```python
from build123d import *

# Parameters (mm, degrees)
SKETCH1_R           = 9.5
SKETCH1_R_2         = 1.6
SKETCH1_R_3         = 0.95
BOSS_EXTRUDE1_DEPTH = 10
SKETCH2_R           = 10
BOSS_EXTRUDE2_DEPTH = 10
SKETCH5_R           = 5.5
CUT_EXTRUDE1_DEPTH  = 1.2


with BuildPart() as part:
    # Sketch1 → Boss-Extrude1 (new body)
    with BuildSketch(Plane.XY):
        Circle(SKETCH1_R)
        Circle(SKETCH1_R_2, mode=Mode.SUBTRACT)
        with Locations((-7.5, 0)):
            Circle(SKETCH1_R_3, mode=Mode.SUBTRACT)
        with Locations((-5.303300859, 5.303300859)):
            Circle(SKETCH1_R_3, mode=Mode.SUBTRACT)
        with Locations((0, 7.5)):
            Circle(SKETCH1_R_3, mode=Mode.SUBTRACT)
        with Locations((5.303300859, 5.303300859)):
            Circle(SKETCH1_R_3, mode=Mode.SUBTRACT)
        with Locations((7.5, 0)):
            Circle(SKETCH1_R_3, mode=Mode.SUBTRACT)
        with Locations((5.303300859, -5.303300859)):
            Circle(SKETCH1_R_3, mode=Mode.SUBTRACT)
        with Locations((0, -7.5)):
            Circle(SKETCH1_R_3, mode=Mode.SUBTRACT)
        with Locations((-5.303300859, -5.303300859)):
            Circle(SKETCH1_R_3, mode=Mode.SUBTRACT)
    extrude(amount=BOSS_EXTRUDE1_DEPTH)

    # Sketch2 → Boss-Extrude2 (add)
    with BuildSketch(Plane.XY.offset(10)):
        with Locations(Location((-2, 0, 0), (0, 0, 69.894490212))):
            Circle(SKETCH2_R)
    extrude(amount=BOSS_EXTRUDE2_DEPTH)

    # Sketch5 → Cut-Extrude1 (cut)
    with BuildSketch(Plane(origin=(0, 0, 0), x_dir=(-1, 0, 0), z_dir=(0, 0, -1))):
        Circle(SKETCH5_R)
    extrude(amount=-CUT_EXTRUDE1_DEPTH, mode=Mode.SUBTRACT)


solid = part.part
```
The listing builds one solid part. Answer for the finished solid, in the listing's coordinates (mm). A direction names the side the tool comes from. Round coordinates to 2 decimals unless told otherwise and drop trailing zeros. Order: outer loops, then holes, each group sorted by start corner. A loop starts at its lowest first (then second) coordinate and runs counter-clockwise, first axis right, second up. Notation, with made-up numbers: (18.5, 15.25) -> (30.5, 15.25) arc R16 ccw to (30.5, 36.25) -> close; hole circle Ø11 at (32.5, 74). An arc over 180 degrees is marked (long way). Answer as CSV lines item,"result".
Q1. Consider line 1 (Y direction, x = 0, z = 6); line 2 (X direction, y = -4.75, z = 4.25); line 3 (X direction, y = -0.75, z = 6.5). Determine where each line is inside the solid, lowest interval first. Write a range as from..to.
Computed values:
line 1,"y = -9.5..-8.45, -6.55..-1.6, 1.6..6.55, 8.45..9.5"
line 2,"x = -8.23..-6.08, -4.53..4.53, 6.08..8.23"
line 3,"x = -9.47..-8.08, -6.92..-1.41, 1.41..6.92, 8.08..9.47"
Q2. Given pin 1 (0.9 mm diameter, centred on x = -7.5, y = 0, fed in from -Z); pin 2 (1 mm diameter, centred on x = -2.5, z = 2.5, fed in from +Y); pin 3 (4 mm diameter, centred on y = -3, z = 10, fed in from -X), each flat-ended and moving along its own axis, determine where each tip first touches the part or whether it passes through.
Computed values:
pin 1,"stops at z = 10"
pin 2,"stops at y = 9.29"
pin 3,"stops at x = -11.95"
Q3. A cutting plane is placed at C-C on x = 2.25. Determine the outline of the cut face in (y, z).
Computed values:
outline,"(-9.23, 0) -> (-5.02, 0) -> (-5.02, 1.2) -> (5.02, 1.2) -> (5.02, 0) -> (9.23, 0) -> (9.23, 10) -> (9.05, 10) -> (9.05, 20) -> (-9.05, 20) -> (-9.05, 10) -> (-9.23, 10) -> close"
Q4. For a pull along Y with two mould halves and no side action, classify faces 1 (the cylindrical face through (-1.27, -0.97, 5.54)), 2 (the flat face through (-10, 0, 10)), 3 (the cylindrical face through (0.986, -9.544, 14.93)) as +Y half, -Y half, draft (parallel to the pull), parting line (faces both ways), or undercut.
Computed values:
face 1,"undercut"
face 2,"draft"
face 3,"parting line"
Q5. A cutting plane is placed at A-A on y = 0. Determine the outline of the cut face in (x, z).
Computed values:
outline,"(-12, 10) -> (-9.5, 10) -> (-9.5, 0) -> (-8.45, 0) -> (-8.45, 10) -> (-6.55, 10) -> (-6.55, 0) -> (-5.5, 0) -> (-5.5, 1.2) -> (-1.6, 1.2) -> (-1.6, 10) -> (1.6, 10) -> (1.6, 1.2) -> (5.5, 1.2) -> (5.5, 0) -> (6.55, 0) -> (6.55, 10) -> (8, 10) -> (8, 20) -> (-12, 20) -> close; (8.45, 0) -> (9.5, 0) -> (9.5, 10) -> (8.45, 10) -> close"
Q6. A cutting plane is placed at B-B on z = 5. Give the number of separate pieces and of enclosed holes in the cut face, plus the area to 3 significant figures.
Computed values:
separate pieces,"1"
enclosed holes,"9"
area,"253 mm^2"
Q7. Which of the six approach directions +Z, -Z, +X, -X, +Y, -Y give full straight-line access (tool end or side, diameter ignored) to faces 4 (the flat face through (8.4, 0.7, 10)), 5 (the flat face through (4, -4, 0)), 6 (the cylindrical face through (-8.45, 0.04, 4.93))?
Computed values:
face 4,"+Z, +X"
face 5,"-Z, +X, -X, +Y, -Y"
face 6,"-Z"
Q8. A cutting plane is placed at D-D on y = -7.5. Determine the outline of the cut face in (x, z).
Computed values:
outline,"(-8.61, 10) -> (-5.83, 10) -> (-5.83, 0) -> (-0.95, 0) -> (-0.95, 10) -> (0.95, 10) -> (0.95, 0) -> (5.83, 0) -> (5.83, 10) -> (4.61, 10) -> (4.61, 20) -> (-8.61, 20) -> close"
